The figure shows three views and two pictorial views of one solid part (mm, origin at its lowest corner). Answer the questions. A direction names the side the tool comes from. Coordinates: 2 decimals unless noted, no trailing zeros. Write each loop counter-clockwise with the first axis right and the second up, starting at its lowest first coordinate (ties: lowest second). Pieces come first, ordered by that corner, then holes.
Item 1: Each of these flat-tipped pins is pushed along its axis until it touches: P1, Ø1.5, axis at x = 419.5, z = 18, coming from the +Y side; P2, Ø6, axis at y = 34.5, z = 14, coming from the -X side; P3, Ø3, axis at y = 52, z = 17, coming from the +X side. Where does it stop, or does it pass through?
Item 2: Section B-B (y = 77.5) is taken. Give the vertices of the cut face in (x, z), then the cut area to 3 significant figures.
Item 3: A tool of negligible diameter and unlimited length cuts with its end or side. For the marked faces 4 and 5, from which of +Z, -Z, +X, -X, +Y, -Y can it reach the whole face along a straight path? Write none if from no direction.
Item 4: Section A-A (x = 545) is taken. Give the vertices of the cut face in (y, z), then the cut area to 3 significant figures.
Item 5: Section C-C (y = 39.5) is taken. Give the vertices of the cut face in (x, z), then the cut area to 3 significant figures.
Item 6: Straight lines are drawn through the part: probe 1 along Z at (x, y) = (545, 208.5); probe 2 along X at (y, z) = (194.5, 15); probe 3 along X at (y, z) = (207.5, 15). For each, find the intervals that lie inside material, in ascending order.
Item 7: Determine the mould class of the marked faces 1, 2 and 3 for opening direction X: released by +X, released by -X, zero draft, split by the parting line, or undercut.
Item 8: Section D-D (x = 367) is taken. Give the vertices of the cut face in (y, z).
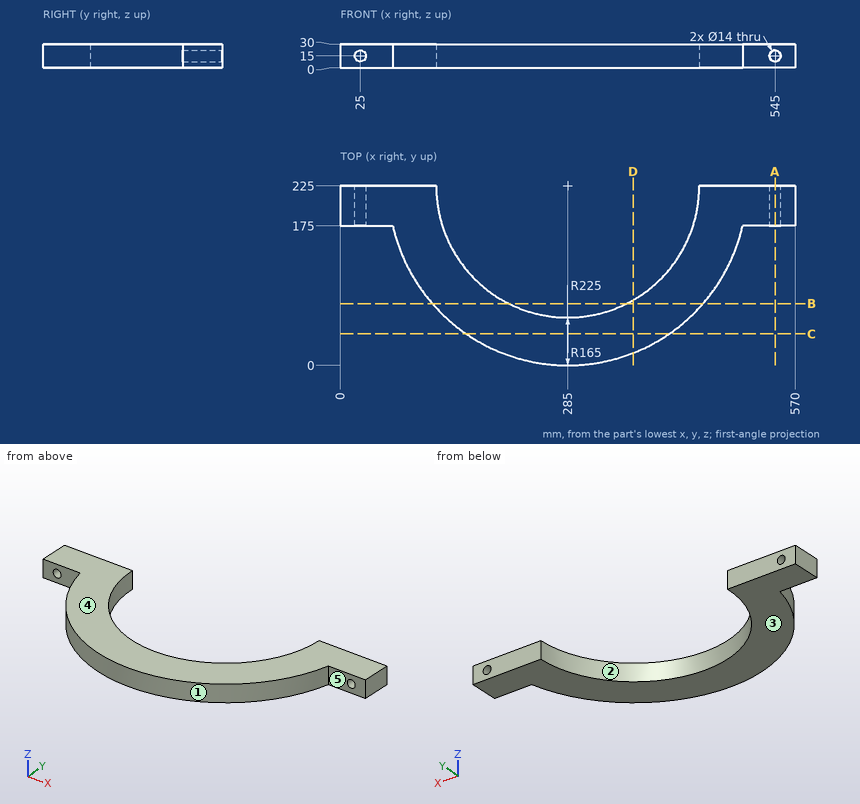
Established:
1. P1: stops at y = 130.49
1. P2: stops at x = 160.63
1. P3: stops at x = 430.65
2. outline: (115.09, 0) - (211.05, 0) - (211.05, 30) - (115.09, 30) - close; (358.95, 0) - (454.91, 0) - (454.91, 30) - (358.95, 30) - close
2. area: 5,760 mm2
3. face 4: +Z, +X, -X, +Y, -Y
3. face 5: +Z, -Z, +X, -Y
4. outline: (175, 0) - (225, 0) - (225, 8) - (175, 8) - close; (175, 22) - (225, 22) - (225, 30) - (175, 30) - close
4. area: 800 mm2
5. outline: (157.66, 0) - (412.34, 0) - (412.34, 30) - (157.66, 30) - close
5. area: 7,640 mm2
6. probe 1: z = 0 to 8, 22 to 30
6. probe 2: x = 0 to 18, 32 to 122.84, 447.16 to 538, 552 to 570
6. probe 3: x = 0 to 18, 32 to 120.93, 449.07 to 538, 552 to 570
7. face 1: split by the parting line
7. face 2: undercut
7. face 3: zero draft
8. outline: (15.47, 0) - (81.82, 0) - (81.82, 30) - (15.47, 30) - close
